Verification items for the finished model (mm, model axes). Face numbers are marked on the shaded views. A direction names the side the tool comes from. Round coordinates to 2 decimals unless told otherwise and drop trailing zeros. Write each loop counter-clockwise with the first axis right and the second up, starting at its lowest first coordinate (ties: lowest second). Pieces come first, ordered by that corner, then holes. Notation, with made-up numbers: M -27.5,-3 L -5.5,-3 A31 cw -5.5,33 Z; hole C 89,-19.5 d10. An arc over 180 degrees is marked long. Use a Markdown table: item, result. Add a question column.
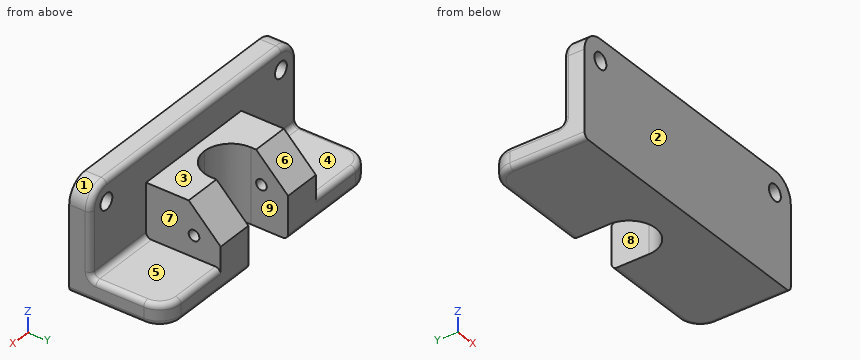
from build123d import *

# Parameters (mm, degrees)
SKETCH1_W                  = 130
SKETCH1_H                  = 100
BOSS_EXTRUDE1_DEPTH        = 20
SKETCH2_W                  = 130
SKETCH2_H                  = 20
BOSS_EXTRUDE2_DEPTH        = 70
FILLET1_R                  = 20
SKETCH3_W                  = 60
SKETCH3_H                  = 70
BOSS_EXTRUDE3_DEPTH        = 50
CUT_EXTRUDE1_DEPTH         = 132.244047484
CHAMFER1_SIZE              = 30
F_10_0_10_DIAMETER_HOLE1_D = 10
F_15_0_15_DIAMETER_HOLE1_D = 15
FILLET2_R                  = 5


with BuildPart() as part:
    # Sketch1 → Boss-Extrude1 (new body)
    with BuildSketch(Plane(origin=(0, 0, 0), x_dir=(1, 0, 0), z_dir=(0, 1, 0))):
        Rectangle(SKETCH1_W, SKETCH1_H)
    extrude(amount=BOSS_EXTRUDE1_DEPTH)

    # Sketch2 → Boss-Extrude2 (add)
    with BuildSketch(Plane(origin=(0, 20, 0), x_dir=(1, 0, 0), z_dir=(0, 1, 0))):
        with Locations((0, 40)):
            Rectangle(SKETCH2_W, SKETCH2_H)
    extrude(amount=BOSS_EXTRUDE2_DEPTH)

    # Fillet1
    fillet1_edges = [part.edges().sort_by_distance(p)[0] for p in [
        (-65, 10, 50),
        (-65, 90, -40),
    ]]
    fillet(fillet1_edges, radius=FILLET1_R)

    # Sketch3 → Boss-Extrude3 (add)
    with BuildSketch(Plane.XY.offset(-30)):
        with Locations((35, 55)):
            Rectangle(SKETCH3_W, SKETCH3_H)
    extrude(amount=BOSS_EXTRUDE3_DEPTH)

    # Sketch4 → Cut-Extrude1 (cut, through all)
    with BuildSketch(Plane.XY.offset(20)):
        with BuildLine():
            Line((40, 90), (40, 55))
            ThreePointArc((40, 55), (47.32233047, 37.32233047), (65, 30))
            Line((65, 30), (65, 90))
            Line((65, 90), (40, 90))
        make_face()
    extrude(amount=-CUT_EXTRUDE1_DEPTH, mode=Mode.SUBTRACT)

    # Chamfer1
    chamfer1_edges = [part.edges().sort_by_distance(p)[0] for p in [
        (22.5, 90, 20),
    ]]
    chamfer(chamfer1_edges, length=CHAMFER1_SIZE)

    # Ø10.0 (10) Diameter Hole1 (through all)
    with Locations(Plane.ZY.offset(-5)):
        with Locations((-10, 65)):
            Hole(F_10_0_10_DIAMETER_HOLE1_D / 2)

    # Ø15.0 (15) Diameter Hole1 (through all)
    with Locations(Plane(origin=(0, 20, 0), x_dir=(1, 0, 0), z_dir=(0, 1, 0))):
        with Locations((-45, -30)):
            Hole(F_15_0_15_DIAMETER_HOLE1_D / 2)

    # Fillet2
    fillet2_edges = [part.edges().sort_by_distance(p)[0] for p in [
        (-65, 20, 0),
        (10, 20, 50),
        (-65, 35, -50),
        (-2.5, 90, -50),
        (-20, 90, -30),
        (-65, 45, -30),
        (-59.142135624, 20, 44.142135624),
        (-59.142135624, 84.142135624, -50),
        (-59.142135624, 84.142135624, -30),
        (-30, 20, -30),
    ]]
    fillet(fillet2_edges, radius=FILLET2_R)

    # 鏡射1: part across plane


with BuildPart() as part_1:
    add(part.part)
    add(part.part.mirror(Plane(origin=(65, 20, 50), x_dir=(0, 0, 1), z_dir=(-1, 0, 0))))


solid = part_1.part
1. Release check for a two-part mould opening along X. For the marked faces 6, 7, 8 and 9 record: +X half, -X half, draft (parallel to the pull), parting line (faces both ways), or undercut.
2. Scan lines: line 1 along Z through (x, y) = (-45, 9); line 2 along X through (y, z) = (79.5, -26); line 3 along X through (y, z) = (15.5, 28.5). Record each from-to range of solid material in increasing order. Write a range as from..to.
3. Cross-section at B-B on x = 118.5. Enter the section's corners in (y, z).
4. Depth check by flat-ended pin: pin 1 Ø1 at (x, z) = (-10, -15) entering from +Y; pin 2 Ø4 at (x, z) = (124.5, 34.5) entering from -Y; pin 3 Ø18 at (x, y) = (-15.5, 48.5) entering from +Z; pin 4 Ø9 at (x, z) = (175, 30) entering from +Y. Enter the tip coordinate at first touch or a pass-through.
5. Cross-section at A-A on y = 12. Enter the section's corners in (x, z).
6. Cross-section at D-D on z = 8. Enter the section's corners in (x, y), plus the area to 3 significant figures.
7. Cross-section at C-C on y = 65. Enter the section's corners in (x, z), plus the area to 3 significant figures.
8. Access from +Z, -Z, +X, -X, +Y, -Y to the whole of each face (thin tool, end or side, straight path). Record for the marked faces 1, 2, 3, 4 and 5.
Answer:
| question | item | result |
|---|---|---|
| 1 | face 6 | draft |
| 1 | face 7 | +X half |
| 1 | face 8 | undercut |
| 1 | face 9 | undercut |
| 2 | line 1 | z = -50..22.5, 37.5..50 |
| 2 | line 2 | x = 5..40, 90..125 |
| 2 | line 3 | x = -64.97..-52.35, -37.65..167.65, 182.35..194.97 |
| 3 | outline | M 0,-50 L 85,-50 A5 ccw 90,-45 L 90,-10 L 60,20 L 20,20 L 20,45 A5 ccw 15,50 L 0,50 Z; hole C 65,-10 d10 |
| 4 | pin 1 | stops at y = 20 |
| 4 | pin 2 | stops at y = 0 |
| 4 | pin 3 | stops at z = -30 |
| 4 | pin 4 | passes through |
| 5 | outline | M -65,-45 A5 ccw -60,-50 L 190,-50 A5 ccw 195,-45 L 195,30 A20 ccw 175,50 L -45,50 A20 ccw -65,30 Z; hole C -45,30 d15; hole C 175,30 d15 |
| 6 | outline | M -65,0 L 195,0 L 195,15 A5 ccw 190,20 L 125,20 L 125,72 L 90,72 L 90,55 A25 cw 40,55 L 40,72 L 5,72 L 5,20 L -60,20 A5 ccw -65,15 Z |
| 6 | area | 9,600 mm^2 |
| 7 | outline | M -65,-45 A5 ccw -60,-50 L 40,-50 L 40,-15 L 5,-15 L 5,-30 L -60,-30 A5 ccw -65,-35 Z; M 5,-5 L 40,-5 L 40,15 L 5,15 Z; M 90,-50 L 190,-50 A5 ccw 195,-45 L 195,-35 A5 ccw 190,-30 L 125,-30 L 125,-15 L 90,-15 Z; M 90,-5 L 125,-5 L 125,15 L 90,15 Z |
| 7 | area | 6,630 mm^2 |
| 8 | face 1 | +Z, +X, +Y, -Y |
| 8 | face 2 | +Z, -Z, +X, -X, -Y |
| 8 | face 3 | +Z, +X, -X, +Y |
| 8 | face 4 | +Z, -X, +Y |
| 8 | face 5 | +Z, +X, +Y |
